The figure shows three views and two pictorial views of one solid part (mm, origin at its lowest corner). Answer the questions. A direction names the side the tool comes from. Give positions to 0.01 mm unless a question says otherwise; leave off trailing zeros. Loops run counter-clockwise (first coordinate to the right, second up) from the corner with the lowest first, then second, coordinate; pieces in that order, holes last. Notation, with made-up numbers: (86.25, 2) - (103.25, 2) arc R27 ccw to (103.25, 31) - close; hole circle Ø11 at (72.5, 18.5). An arc over 180 degrees is marked (long way). Write item = value, one per line.
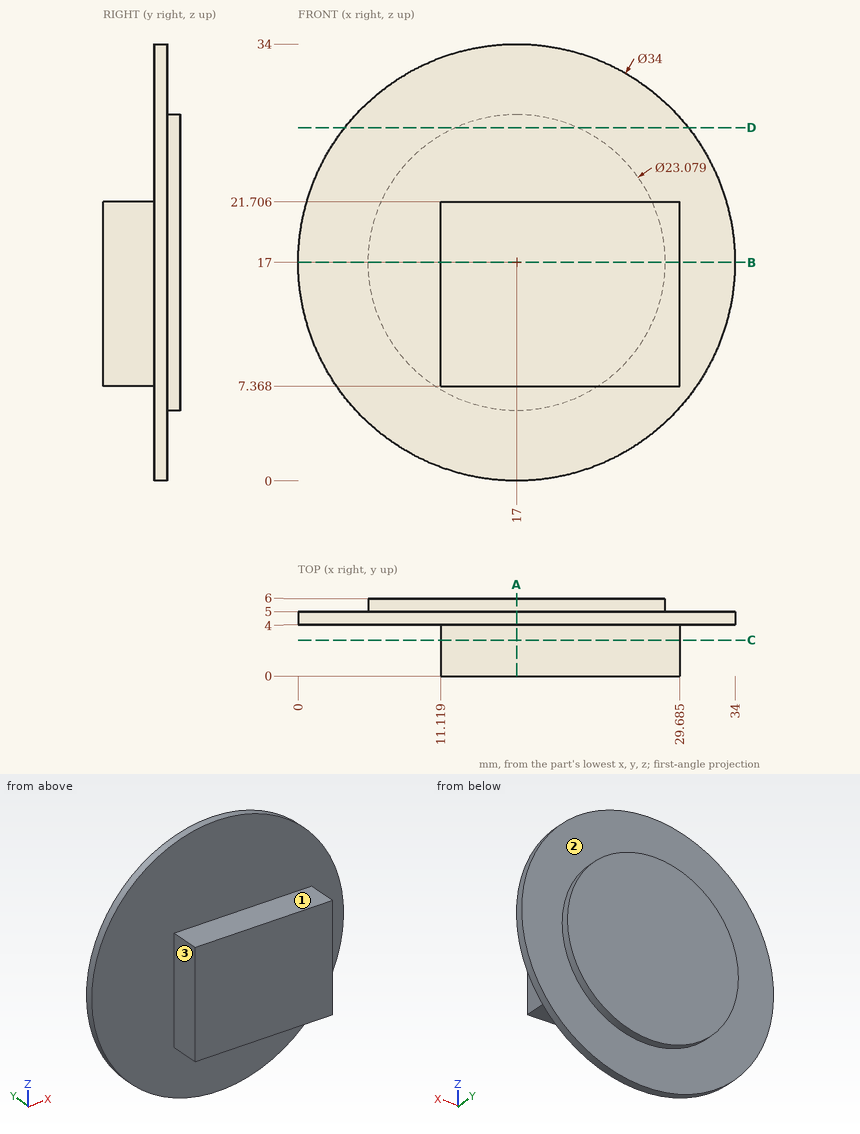
1) A cutting plane is placed at D-D on z = 27.5. Determine the outline of the cut face in (x, y).
Output:
outline = (3.63, 4) - (30.37, 4) - (30.37, 5) - (21.79, 5) - (21.79, 6) - (12.21, 6) - (12.21, 5) - (3.63, 5) - close
2) A cutting plane is placed at A-A on x = 17. Determine the outline of the cut face in (y, z).
Output:
outline = (0, 7.37) - (4, 7.37) - (4, 0) - (5, 0) - (5, 5.46) - (6, 5.46) - (6, 28.54) - (5, 28.54) - (5, 34) - (4, 34) - (4, 21.71) - (0, 21.71) - close
3) Each of these flat-tipped pins is pushed along its axis until it touches: P1, Ø1.2, axis at y = 1.5, z = 14.5, coming from the -X side; P2, Ø3, axis at x = 21.5, y = 2, coming from the -Z side; P3, Ø1.2, axis at y = 1.5, z = 12.5, coming from the +X side (3 decimals). Where does it stop, or does it pass through?
Output:
P1 = 11.12
P2 = 7.37
P3 = 29.685
4) Find the intervals of material crossed by probe 1 along Y at (x, z) = (23, 31); probe 2 along Z at (x, y) = (20.5, 2.7); probe 3 along Y at (x, z) = (12, 26.5), in increasing order.
Output:
probe_1 = 4 to 5
probe_2 = 7.37 to 21.71
probe_3 = 4 to 6
5) A cutting plane is placed at C-C on y = 2.8. Determine the outline of the cut face in (x, z) (1 decimal).
Output:
outline = (11.1, 7.4) - (29.7, 7.4) - (29.7, 21.7) - (11.1, 21.7) - close
6) A tool of negligible diameter and unlimited length cuts with its end or side. For the marked faces 1, 2 and 3, from which of +Z, -Z, +X, -X, +Y, -Y can it reach the whole face along a straight path? Write none if from no direction.
Output:
face_1 = +Z, +X, -X, -Y
face_2 = +Y
face_3 = +Z, -Z, -X, -Y
7) A cutting plane is placed at B-B on z = 17. Determine the outline of the cut face in (x, y) (1 decimal).
Output:
outline = (0, 4) - (11.1, 4) - (11.1, 0) - (29.7, 0) - (29.7, 4) - (34, 4) - (34, 5) - (28.5, 5) - (28.5, 6) - (5.5, 6) - (5.5, 5) - (0, 5) - close
